Check sheet for the drawn part. Datum: minimum x, y, z corner. Units: mm. Round coordinates to 2 decimals unless told otherwise and drop trailing zeros. Write each loop counter-clockwise with the first axis right and the second up, starting at its lowest first coordinate (ties: lowest second). Pieces come first, ordered by that corner, then holes.
Item 1: Material ranges on line 1 (X direction, y = 2.25, z = 6), recorded low to high.
Item 2: Go/stop test with flat-tipped pins: pin 1 Ø1.5 at (y, z) = (2, 68) entering from +X; pin 2 Ø1 at (x, y) = (67, 2.5) entering from +Z; pin 3 Ø1.5 at (y, z) = (1.5, 124.5) entering from -X. Record where each tip stops, or that it passes through.
Item 3: Cross-section at B-B on x = 23.5. Enter the section's corners in (y, z).
Item 4: Cross-section at A-A on z = 81. Enter the section's corners in (x, y), plus the area to 3 significant figures.
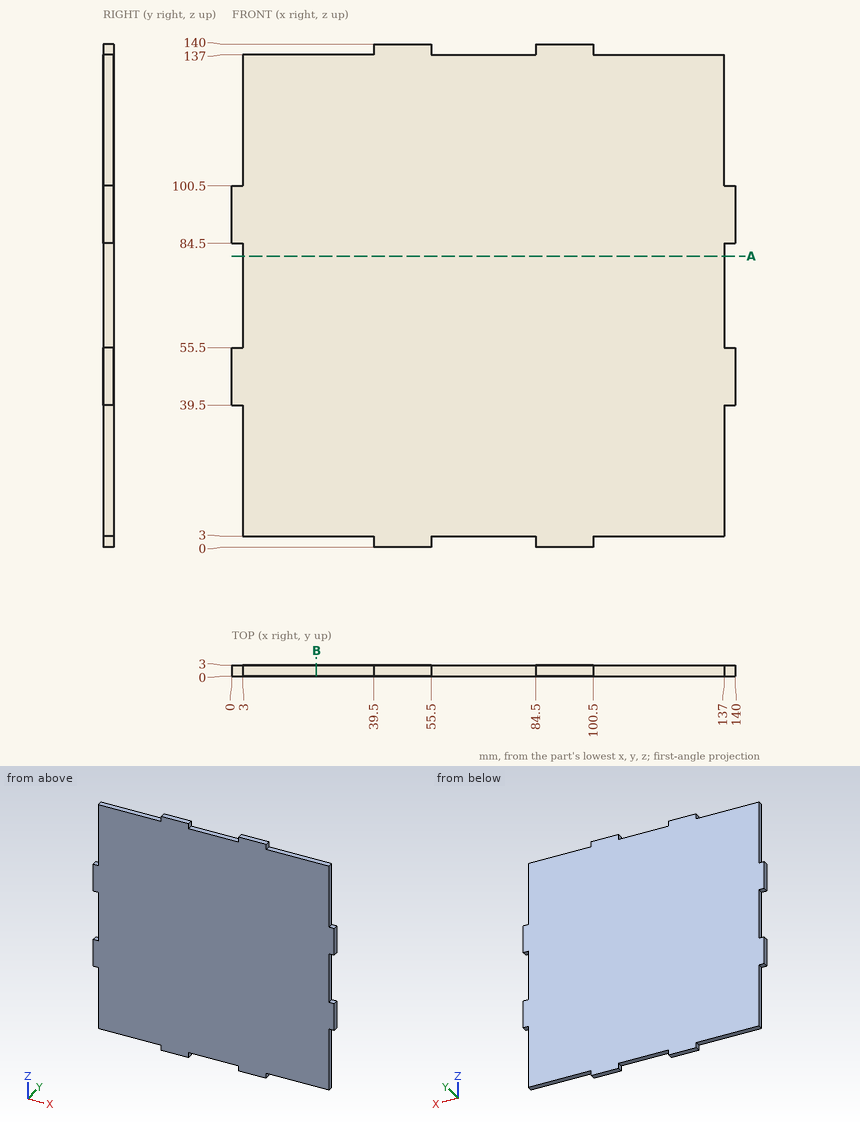
Response values:
1. line 1: x = 3 to 137
2. pin 1: stops at x = 137
2. pin 2: stops at z = 137
2. pin 3: stops at x = 3
3. outline: (0, 3) - (3, 3) - (3, 137) - (0, 137) - close
4. outline: (3, 0) - (137, 0) - (137, 3) - (3, 3) - close
4. area: 402 mm2
